Here's how the part is built. I have some questions about the finished solid (model axes, mm). Coordinates: 2 decimals unless noted, no trailing zeros. Write each loop counter-clockwise with the first axis right and the second up, starting at its lowest first coordinate (ties: lowest second). Pieces come first, ordered by that corner, then holes.
```python
from build123d import *

# Parameters (mm, degrees)
BOSS_EXTRUDE1_DEPTH      = 1.5875
BOSS_EXTRUDE1_DEPTH_BACK = 1.5875
SKETCH1_W                = 600
SKETCH1_H                = 600
SKETCH1_R                = 2.6
SKETCH1_R_2              = 26.67


with BuildPart() as part:
    # Sketch1 → Boss-Extrude1 (new, two sides: drawn at the far end of the back side and taken through both)
    with BuildSketch(Plane(origin=(0, 0, 0), x_dir=(1, 0, 0), z_dir=(0, 1, 0)).offset(-BOSS_EXTRUDE1_DEPTH_BACK)):
        Rectangle(SKETCH1_W, SKETCH1_H)
        with Locations(Location((-290, 290, 0), (0, 0, 270))):
            Circle(SKETCH1_R, mode=Mode.SUBTRACT)
        with Locations(Location((290, 290, 0), (0, 0, 90))):
            Circle(SKETCH1_R, mode=Mode.SUBTRACT)
        with Locations(Location((290, -290, 0), (0, 0, 270))):
            Circle(SKETCH1_R, mode=Mode.SUBTRACT)
        with Locations(Location((-290, -290, 0), (0, 0, 90))):
            Circle(SKETCH1_R, mode=Mode.SUBTRACT)
        with Locations(Location((0, 0, 0), (0, 0, 270))):
            Circle(SKETCH1_R_2, mode=Mode.SUBTRACT)
        with Locations(Location((100, 0, 0), (0, 0, 270))):
            Circle(SKETCH1_R_2, mode=Mode.SUBTRACT)
        with Locations(Location((200, 0, 0), (0, 0, 270))):
            Circle(SKETCH1_R_2, mode=Mode.SUBTRACT)
        with Locations(Location((100, 100, 0), (0, 0, 270))):
            Circle(SKETCH1_R_2, mode=Mode.SUBTRACT)
        with Locations(Location((200, 100, 0), (0, 0, 270))):
            Circle(SKETCH1_R_2, mode=Mode.SUBTRACT)
        with Locations(Location((100, 200, 0), (0, 0, 270))):
            Circle(SKETCH1_R_2, mode=Mode.SUBTRACT)
        with Locations(Location((200, 200, 0), (0, 0, 270))):
            Circle(SKETCH1_R_2, mode=Mode.SUBTRACT)
        with Locations(Location((0, 100, 0), (0, 0, 270))):
            Circle(SKETCH1_R_2, mode=Mode.SUBTRACT)
        with Locations(Location((0, 200, 0), (0, 0, 270))):
            Circle(SKETCH1_R_2, mode=Mode.SUBTRACT)
        with Locations(Location((-100, 0, 0), (0, 0, 270))):
            Circle(SKETCH1_R_2, mode=Mode.SUBTRACT)
        with Locations(Location((-200, 0, 0), (0, 0, 270))):
            Circle(SKETCH1_R_2, mode=Mode.SUBTRACT)
        with Locations(Location((-100, -100, 0), (0, 0, 270))):
            Circle(SKETCH1_R_2, mode=Mode.SUBTRACT)
        with Locations(Location((-200, -100, 0), (0, 0, 270))):
            Circle(SKETCH1_R_2, mode=Mode.SUBTRACT)
        with Locations(Location((-100, -200, 0), (0, 0, 270))):
            Circle(SKETCH1_R_2, mode=Mode.SUBTRACT)
        with Locations(Location((-200, -200, 0), (0, 0, 270))):
            Circle(SKETCH1_R_2, mode=Mode.SUBTRACT)
        with Locations(Location((0, -100, 0), (0, 0, 270))):
            Circle(SKETCH1_R_2, mode=Mode.SUBTRACT)
        with Locations(Location((0, -200, 0), (0, 0, 270))):
            Circle(SKETCH1_R_2, mode=Mode.SUBTRACT)
        with Locations(Location((200, -200, 0), (0, 0, 90))):
            Circle(SKETCH1_R_2, mode=Mode.SUBTRACT)
        with Locations(Location((100, -200, 0), (0, 0, 90))):
            Circle(SKETCH1_R_2, mode=Mode.SUBTRACT)
        with Locations(Location((200, -100, 0), (0, 0, 90))):
            Circle(SKETCH1_R_2, mode=Mode.SUBTRACT)
        with Locations(Location((100, -100, 0), (0, 0, 90))):
            Circle(SKETCH1_R_2, mode=Mode.SUBTRACT)
        with Locations(Location((-200, 200, 0), (0, 0, 90))):
            Circle(SKETCH1_R_2, mode=Mode.SUBTRACT)
        with Locations(Location((-100, 200, 0), (0, 0, 90))):
            Circle(SKETCH1_R_2, mode=Mode.SUBTRACT)
        with Locations(Location((-200, 100, 0), (0, 0, 90))):
            Circle(SKETCH1_R_2, mode=Mode.SUBTRACT)
        with Locations(Location((-100, 100, 0), (0, 0, 90))):
            Circle(SKETCH1_R_2, mode=Mode.SUBTRACT)
    extrude(amount=BOSS_EXTRUDE1_DEPTH + BOSS_EXTRUDE1_DEPTH_BACK)


solid = part.part
```
1) Imagine slicing it at A-A on x = -200. Please give me the cut outline in (y, z).
Values follow:
outline: (-1.59, -300) - (1.59, -300) - (1.59, -226.67) - (-1.59, -226.67) - close; (-1.59, -173.33) - (1.59, -173.33) - (1.59, -126.67) - (-1.59, -126.67) - close; (-1.59, -73.33) - (1.59, -73.33) - (1.59, -26.67) - (-1.59, -26.67) - close; (-1.59, 26.67) - (1.59, 26.67) - (1.59, 73.33) - (-1.59, 73.33) - close; (-1.59, 126.67) - (1.59, 126.67) - (1.59, 173.33) - (-1.59, 173.33) - close; (-1.59, 226.67) - (1.59, 226.67) - (1.59, 300) - (-1.59, 300) - close
2) Imagine slicing it at B-B on z = 200. Please give me the cut outline in (x, y).
Values follow:
outline: (-300, -1.59) - (-226.67, -1.59) - (-226.67, 1.59) - (-300, 1.59) - close; (-173.33, -1.59) - (-126.67, -1.59) - (-126.67, 1.59) - (-173.33, 1.59) - close; (-73.33, -1.59) - (-26.67, -1.59) - (-26.67, 1.59) - (-73.33, 1.59) - close; (26.67, -1.59) - (73.33, -1.59) - (73.33, 1.59) - (26.67, 1.59) - close; (126.67, -1.59) - (173.33, -1.59) - (173.33, 1.59) - (126.67, 1.59) - close; (226.67, -1.59) - (300, -1.59) - (300, 1.59) - (226.67, 1.59) - close
3) We'd pull the mould along X, two halves only. Please class faces 1 (the face through (-4, 1.588, -71)), 2 (the face through (123.66, -0.02, 87.69)): pulls with the +X half, pulls with the -X half, needs draft (parallel to the pull), parting line crosses it, or undercut.
Values follow:
face 1: needs draft
face 2: undercut
4) I need wall thicknesses on probe 1 along X at (y, z) = (-0.85, -200); probe 2 along Z at (x, y) = (290, 0.05); probe 3 along Z at (x, y) = (18.5, 0). Which ranges of each line are inside material? Lowest first, please.
Values follow:
probe 1: x = -300 to -226.67, -173.33 to -126.67, -73.33 to -26.67, 26.67 to 73.33, 126.67 to 173.33, 226.67 to 300
probe 2: z = -300 to -292.6, -287.4 to 287.4, 292.6 to 300
probe 3: z = -300 to -219.21, -180.79 to -119.21, -80.79 to -19.21, 19.21 to 80.79, 119.21 to 180.79, 219.21 to 300
5) Imagine slicing it at C-C on y = 0.7. Count the separate pieces of the cut face and the enclosed holes in it, then the cut area to 3 significant figures.
Values follow:
separate pieces: 1
enclosed holes: 29
area: 304,000 mm2
